Part model, mm, in its own coordinate system. Face numbers are marked on the shaded views. Round coordinates to 2 decimals unless told otherwise and drop trailing zeros. Write each loop counter-clockwise with the first axis right and the second up, starting at its lowest first coordinate (ties: lowest second). Pieces come first, ordered by that corner, then holes. Notation, with made-up numbers: (11, 51) -> (32, 51) arc R22 ccw to (32, 59) -> close; hole circle Ø1 at (-3, 47.5). An arc over 180 degrees is marked (long way). Use CSV: the item, a comma, the result in double quotes. Start each with the question number.
(1) Drop flat-ended pins along their axis: pin 1 (4 mm diameter, centred on x = 40, y = 4.5, fed in from +Z); pin 2 (3 mm diameter, centred on x = 17, z = 3.5, fed in from -Y); pin 3 (1.5 mm diameter, centred on x = 14, z = 4.5, fed in from -Y). Give the stop position or say it passes through.
(2) Two-plate mould, pull along X, no slides. Class the marked faces 1, 2 and 3: released by +X, released by -X, zero draft, split by the parting line, or undercut.
(3) Probe line 1 (Y direction, x = 21, z = -3); line 2 (Y direction, x = 28.5, z = 0); line 3 (Z direction, x = 11.5, y = -0.5). List the from-to ranges inside material, lowest first. Write a range as [from, to].
(4) Saw through at A-A (z = 0). Give the cut face in (x, y).
(5) Saw through at C-C (x = 17). Give the cut face in (y, z).
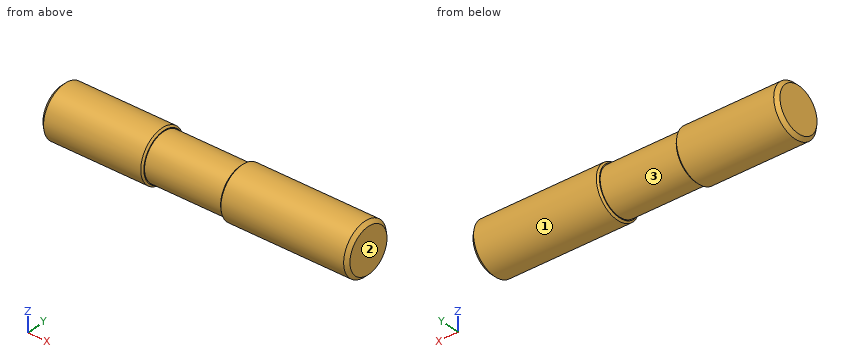
Autodesk Inventor part; units mm, degrees
ref_plane "Work Plane1" through (24, 0, 0) normal (1, 0, 0) x (0, 1, 0)
ref_plane "YZ Plane" through (0, 0, 0) normal (1, 0, 0) x (0, 1, 0)
ref_plane "XZ Plane" through (0, 0, 0) normal (0, 1, 0) x (-1, 0, 0)
sketch "Sketch1" plane through (0, 0, 0) normal (0, 0, 1) x (1, 0, 0)
  line L0 (0, 0) -> (0, 6)
  line L1 (0, 6) -> (24, 6)
  line L2 (24, 6) -> (24, 5.4145)
  line L3 (24, 5.4145) -> (42, 5.4145)
  line L4 (42, 5.4145) -> (42, 6)
  line L5 (42, 6) -> (72, 6)
  line L6 (72, 6) -> (72, 0)
  line L7 (72, 0) -> (0, 0)
  dimension "d1" = 12
  dimension "d3" = 10.829
  dimension "d4" = 24
  dimension "d5" = 48
  dimension "d6" = 30
revolve "Вращение1" add sketch "Sketch1" angle 360 about axis through (72, 0, 0) along (-1, 0, 0)
thread "Резьба1"
thread "Резьба2"
chamfer "Фаска1" distance 0.8 angle 45 2 edges at (0, -6, 0) (72, -6, 0)
chamfer "Фаска2" distance 0.4 angle 45 2 edges at (24, -6, 0) (42, -6, 0)
ref_plane "Work Plane1" through (24, 0, 0) normal (1, 0, 0) x (0, 1, 0)
sketch "Sketch2" plane through (24, 0, 0) normal (1, 0, 0) x (0, 1, 0)
  circle A0 centre (0, 0) radius 6
  point P0 (0, 0)
  dimension "d35" = 12
boundary_patch "Участок поверхности1"
equation "\"d8\" = d4"
equation "\"d29\" = b"
equation "\"d31\" = C_"
equation "\"d37\" = C2_"
equation "\"d1\" = d"
equation "\"d3\" = d2"
equation "\"d4\" = b1"
equation "\"d5\" = L"
equation "\"d6\" = b"
equation "\"d35\" = d"
equation "\"C_\" = 0.8"
equation "\"d\" = 12"
equation "\"d2\" = 10.829"
equation "\"b1\" = 24"
equation "\"L\" = 48"
equation "\"b\" = 30"
equation "\"d34\" = -b1"
equation "\"C2_\" = 0.4"
equation "\"Grip_Length\" = 18"
properties part number "Шпилька 2 M12-6g×48 ГОСТ 22038-76" material "Сталь, мягкая"
Answers:
1,pin 1,"stops at z = 4.8"
1,pin 2,"stops at y = -5.66"
1,pin 3,"stops at y = -4.68"
2,face 1,"zero draft"
2,face 2,"released by +X"
2,face 3,"undercut"
3,line 1,"y = [-5.2, 5.2]"
3,line 2,"y = [-5.41, 5.41]"
3,line 3,"z = [-5.98, 5.98]"
4,outline,"(0, -5.2) -> (0.8, -6) -> (23.6, -6) -> (24, -5.6) -> (24, -5.41) -> (42, -5.41) -> (42, -5.6) -> (42.4, -6) -> (71.2, -6) -> (72, -5.2) -> (72, 5.2) -> (71.2, 6) -> (42.4, 6) -> (42, 5.6) -> (42, 5.41) -> (24, 5.41) -> (24, 5.6) -> (23.6, 6) -> (0.8, 6) -> (0, 5.2) -> close"
5,outline,"circle Ø12 at (0, 0)"
